Autodesk Inventor part; units mm, degrees
ref_plane "YZ Plane" through (0, 0, 0) normal (1, 0, 0) x (0, 1, 0)
ref_plane "XZ Plane" through (0, 0, 0) normal (0, 1, 0) x (-1, 0, 0)
ref_plane "XY Plane" through (0, 0, 0) normal (0, 0, 1) x (1, 0, 0)
sketch "スケッチ1" plane through (0, 0, 0) normal (0, 1, 0) x (-1, 0, 0)
  line L0 (0, 0) -> (47.5, 0)
  line L1 (47.5, 0) -> (47.5, -120)
  line L2 (47.5, -120) -> (0, -120)
  line L3 (0, -120) -> (0, 0)
  dimension "d0" = 47.5
  dimension "d1" = 120
extrude "押し出し1" add sketch "スケッチ1" along normal blind 10
ref_plane "作業平面1" through (0, 10, 0) normal (0, 1, 0) x (1, 0, 0)
sketch "スケッチ2" plane through (0, 10, 0) normal (0, 1, 0) x (1, 0, 0)
  line L0 (0, 120) -> (-47.5, 120)
  line L1 (0, 0) -> (0, 120)
  line L2 (-47.5, 120) -> (0, 120)
  line L3 (0, 120) -> (0, 96)
  line L4 (0, 96) -> (-47.5, 96)
  line L5 (-47.5, 96) -> (-47.5, 120)
  line L6 (-47.5, 120) -> (-47.5, 0)
  line L7 (0, 0) -> (-47.5, 0)
  line L8 (-47.5, 0) -> (-47.5, 24)
  line L9 (-47.5, 24) -> (0, 24)
  line L10 (0, 24) -> (0, 0)
  point P0 (0, 24)
  dimension "d5" = 24
  dimension "d6" = 24
  dimension "d7" = 72
extrude "押し出し2" cut sketch "スケッチ2" against normal blind 4 contours L1 L4 L5 L0 | L1 L7 L6 L9
ref_plane "作業平面2" through (0, 0, 0) normal (0, -1, 0) x (1, 0, 0)
sketch "スケッチ3" plane through (0, 0, 0) normal (0, -1, 0) x (1, 0, 0)
  line L0 (-47.5, 0) -> (0, 0)
  line L1 (0, -120) -> (-47.5, -120)
  line L2 (-47.5, -120) -> (-47.5, 0)
  line L3 (0, 0) -> (0, -120)
  point P0 (-39.5, -12)
  point P1 (-8, -12)
  point P2 (-39.5, -108)
  point P3 (-8, -108)
  dimension "d11" = 12
  dimension "d12" = 12
  dimension "d13" = 12
  dimension "d14" = 12
  dimension "d15" = 8
  dimension "d16" = 8
  dimension "d17" = 8
  dimension "d18" = 8
hole "穴1" at (-39.5, 0, -12) at (-8, 0, -12) at (-39.5, 0, -108) at (-8, 0, -108) direction (0, 1, 0) diameter 5.8 depth 7
sketch "スケッチ4" plane through (0, 0, 0) normal (0, -1, 0) x (1, 0, 0)
  circle A0 centre (-8, -12) radius 2.9
  circle A1 centre (-8, -12) radius 4.5
  circle A2 centre (-39.5, -12) radius 2.9
  circle A3 centre (-39.5, -12) radius 4.5
  circle A4 centre (-39.5, -108) radius 2.9
  circle A5 centre (-39.5, -108) radius 4.5
  circle A6 centre (-8, -108) radius 2.9
  circle A7 centre (-8, -108) radius 4.5
  point P0 (0, 0)
  dimension "d26" = 9
  dimension "d27" = 9
  dimension "d28" = 9
  dimension "d29" = 9
extrude "押し出し3" cut sketch "スケッチ4" against normal blind 3
properties part number "motor_rot_born2"
For this review, take the finished solid that the model builds, in its own axes (mm). A direction names the side the tool comes from. Give positions to 0.01 mm unless a question says otherwise; leave off trailing zeros. Loops run counter-clockwise (first coordinate to the right, second up) from the corner with the lowest first, then second, coordinate; pieces in that order, holes last. Notation, with made-up numbers: M 54.25,-3.5 L 89.25,-3.5 A15 cw 89.25,12.5 Z; hole C 48.25,14.25 d1. An arc over 180 degrees is marked long. One line per item, written item: value. Start each with the question number.
Q1. Clearance check with flat-ended pins moving along their axes: pin 1 Ø7 at (x, z) = (-40.5, -12.5) entering from -Y; pin 2 Ø7 at (x, z) = (-22.5, -17) entering from +Y; pin 3 Ø2.5 at (x, z) = (-37.5, -108.5) entering from -Y; pin 4 Ø2 at (x, y) = (-26.5, 8.5) entering from +Z. State where each tip first meets the part, or that it passes through.
Q2. For L1, parallel to Z at x = -8, y = 5.25; L2, parallel to Z at x = -8, y = 2.4; L3, parallel to Z at x = -26.5, y = 7.25, list the stretches that pass through material, from the lowest coordinate up.
Q3. Draft analysis for pull direction X (two halves, no side actions). For faces 5 (the face through (0, 4, -61)), 6 (the face through (-5.581, 1.479, -104.206)), 7 (the face through (-23, 10, -59)), state which applies: released by +X, released by -X, zero draft, split by the parting line, or undercut.
Q4. Add section D-D (x = -30). Give the boundary of the cut face in (y, z).
Q5. Machinability: for faces 1 (the face through (-39.6, 4.5, -105.1)), 2 (the face through (-7, 3, -15)), 3 (the face through (-24, 6, -12)), 4 (the face through (-23, 8, -96)), which of the approach directions +Z, -Z, +X, -X, +Y, -Y give a long, thin tool a straight path to every point of the face, cutting with its end or side? Answer none if there is none.
Q6. Add section C-C (y = 4.75). Give the boundary of the cut face in (x, z), and give its area (3 significant figures).
Q7. Add section A-A (z = -12). Give the boundary of the cut face in (x, y), and give its area (3 significant figures).
Q8. Add section B-B (x = -8). Give the boundary of the cut face in (y, z), and give its area (3 significant figures).
Reply:
1. pin 1: y = 0
1. pin 2: y = 6
1. pin 3: y = 3
1. pin 4: z = -24
2. L1: -120 to -110.9, -105.1 to -14.9, -9.1 to 0
2. L2: -120 to -112.5, -103.5 to -16.5, -7.5 to 0
2. L3: -96 to -24
3. face 5: released by +X
3. face 6: undercut
3. face 7: zero draft
4. outline: M 0,-120 L 6,-120 L 6,-96 L 10,-96 L 10,-24 L 6,-24 L 6,0 L 0,0 Z
5. face 1: +Y, -Y
5. face 2: -Y
5. face 3: +Z, +X, -X, +Y
5. face 4: -Z, +X, -X, +Y
6. outline: M -47.5,-120 L 0,-120 L 0,0 L -47.5,0 Z; hole C -39.5,-108 d5.8; hole C -39.5,-12 d5.8; hole C -8,-108 d5.8; hole C -8,-12 d5.8
6. area: 5,590 mm²
7. outline: M -47.5,0 L -44,0 L -44,3 L -42.4,3 L -42.4,6 L -47.5,6 Z; M -36.6,3 L -35,3 L -35,0 L -12.5,0 L -12.5,3 L -10.9,3 L -10.9,6 L -36.6,6 Z; M -5.1,3 L -3.5,3 L -3.5,0 L 0,0 L 0,6 L -5.1,6 Z
7. area: 196 mm²
8. outline: M 0,-120 L 6,-120 L 6,-110.9 L 3,-110.9 L 3,-112.5 L 0,-112.5 Z; M 0,-103.5 L 3,-103.5 L 3,-105.1 L 6,-105.1 L 6,-96 L 10,-96 L 10,-24 L 6,-24 L 6,-14.9 L 3,-14.9 L 3,-16.5 L 0,-16.5 Z; M 0,-7.5 L 3,-7.5 L 3,-9.1 L 6,-9.1 L 6,0 L 0,0 Z
8. area: 919 mm²
